Input: part model. Units: mm. Frame: model coordinates. Face numbers are marked on the shaded views. A direction names the side the tool comes from. Coordinates: 2 decimals unless noted, no trailing zeros. Write each loop counter-clockwise with the first axis right and the second up, starting at its lowest first coordinate (ties: lowest second). Pieces come first, ordered by that corner, then holes. Notation, with made-up numbers: (-22, -3.5) -> (34, -3.5) arc R27 cw to (34, 18.5) -> close; hole circle Ø3 at (25, 78.5). An arc over 180 degrees is marked (long way). One line per question, with ' | ' between items. Start each with the question number.
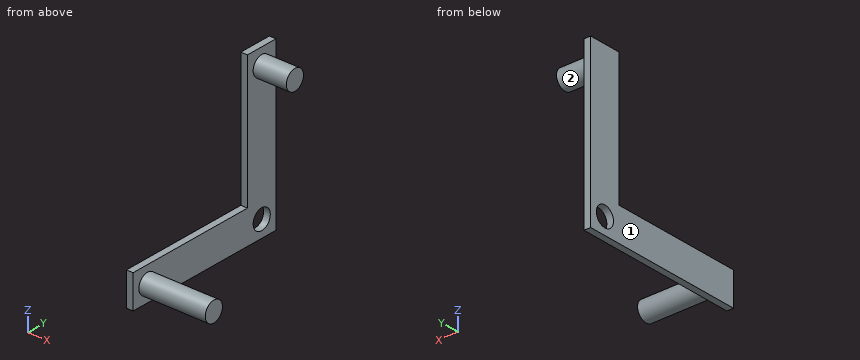
```python
from build123d import *

# Parameters (mm, degrees)
SKETCH1_W           = 10
SKETCH1_H           = 50
BOSS_EXTRUDE1_DEPTH = 2
SKETCH2_R           = 3
CUT_EXTRUDE1_DEPTH  = 2
SKETCH3_R           = 3
BOSS_EXTRUDE2_DEPTH = 20
SKETCH4_W           = 2
SKETCH4_H           = 10
BOSS_EXTRUDE3_DEPTH = 40
SKETCH5_R           = 3
BOSS_EXTRUDE4_DEPTH = 10


with BuildPart() as part:
    # Sketch1 → Boss-Extrude1 (new body)
    with BuildSketch(Plane(origin=(0, 0, 0), x_dir=(0, 0, -1), z_dir=(1, 0, 0))):
        Rectangle(SKETCH1_W, SKETCH1_H)
    extrude(amount=BOSS_EXTRUDE1_DEPTH)

    # Sketch2 → Cut-Extrude1 (cut)
    with BuildSketch(Plane(origin=(2, 0, 0), x_dir=(0, 0, -1), z_dir=(1, 0, 0))):
        with Locations((0, 20)):
            Circle(SKETCH2_R)
    extrude(amount=-CUT_EXTRUDE1_DEPTH, mode=Mode.SUBTRACT)

    # Sketch3 → Boss-Extrude2 (add)
    with BuildSketch(Plane(origin=(2, 0, 0), x_dir=(0, 0, -1), z_dir=(1, 0, 0))):
        with Locations((0, -20)):
            Circle(SKETCH3_R)
    extrude(amount=BOSS_EXTRUDE2_DEPTH)

    # Sketch4 → Boss-Extrude3 (add)
    with BuildSketch(Plane.XY.offset(5)):
        with Locations((1, 20)):
            Rectangle(SKETCH4_W, SKETCH4_H)
    extrude(amount=BOSS_EXTRUDE3_DEPTH)

    # Sketch5 → Boss-Extrude4 (add)
    with BuildSketch(Plane(origin=(2, 0, 0), x_dir=(0, 0, -1), z_dir=(1, 0, 0))):
        with Locations((-40, 20)):
            Circle(SKETCH5_R)
    extrude(amount=BOSS_EXTRUDE4_DEPTH)


solid = part.part
```
1) Section D-D, the plane z = 40. Return loops of the section in (x, y).
2) Section B-B, the plane y = 20. Return loops of the section in (x, z).
3) Section C-C, the plane y = -20. Return loops of the section in (x, z).
4) Ray query, line 1 (Y direction, x = 1.05, z = 0); line 2 (X direction, y = 8, z = 1); line 3 (Z direction, x = 1.5, y = 9). Return the intervals inside material, ascending.
5) First-contact query: P1, Ø0.6, axis at x = 0.5, y = -2.5, coming from the +Z side; P2, Ø6, axis at x = 12, z = 35, coming from the +Y side; P3, Ø5, axis at x = 8, z = 36.5, coming from the +Y side; P4, Ø3, axis at x = 5, y = -2.5, coming from the +Z side. Flat tips, straight axial feed; report the tip coordinate or a pass-through.
6) Section A-A, the plane z = 0. Return loops of the section in (x, y), then the cut area to 3 significant figures.
7) Access query for the marked faces 1 and 2. Directions: +Z, -Z, +X, -X, +Y, -Y. A direction counts if a zero-diameter tool reaches every point of the face in a straight line with its end or side. Return the directions, or none.
Answer block:
1) outline: (0, 15) -> (2, 15) -> (2, 17) -> (12, 17) -> (12, 23) -> (2, 23) -> (2, 25) -> (0, 25) -> close
2) outline: (0, -5) -> (2, -5) -> (2, -3) -> (0, -3) -> close; (0, 3) -> (2, 3) -> (2, 37) -> (12, 37) -> (12, 43) -> (2, 43) -> (2, 45) -> (0, 45) -> close
3) outline: (0, -5) -> (2, -5) -> (2, -3) -> (22, -3) -> (22, 3) -> (2, 3) -> (2, 5) -> (0, 5) -> close
4) line 1: y = -25 to 17, 23 to 25 | line 2: x = 0 to 2 | line 3: z = -5 to 5
5) P1: stops at z = 5 | P2: stops at y = 22.24 | P3: stops at y = 22.83 | P4: passes through
6) outline: (0, -25) -> (2, -25) -> (2, -23) -> (22, -23) -> (22, -17) -> (2, -17) -> (2, 17) -> (0, 17) -> close; (0, 23) -> (2, 23) -> (2, 25) -> (0, 25) -> close | area: 208 mm2
7) face 1: +Z, -Z, -X, +Y, -Y | face 2: +X
